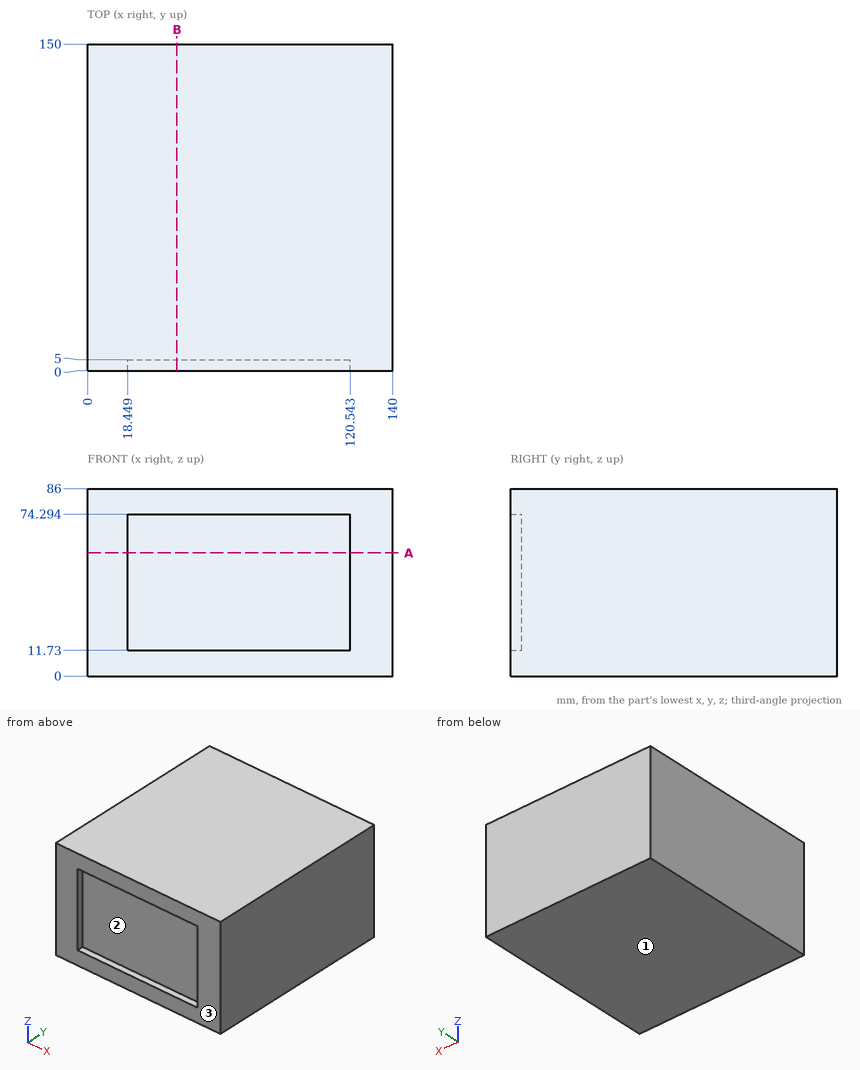
Here's the drawing with two shaded views (mm, measured from the low corner). I have some questions. Coordinates: 2 decimals unless noted, no trailing zeros. Write each loop counter-clockwise with the first axis right and the second up, starting at its lowest first coordinate (ties: lowest second). Pieces come first, ordered by that corner, then holes.
Item 1: If we mould it in two halves opening along Z, with no side actions, what happens to the marked faces 1, 2 and 3? For each: +Z half, -Z half, draft (parallel to the pull), parting line (faces both ways), or undercut.
Item 2: I want a section at A-A on z = 56.5. Write out the boundary of the cut face in (x, y).
Item 3: If I drill on line 1 (Y direction, x = 94, z = 15.5), over which ranges is the centre line in solid material (lowest first)?
Item 4: Will this pin go through, and if not, where does the flat tip stop? pin 1 (8 mm diameter, centred on x = 31.5, z = 39, fed in from -Y).
Item 5: I want a section at B-B on x = 41. Write out the boundary of the cut face in (y, z) (1 decimal), and give its area (3 significant figures).
Findings below:
1. face 1: -Z half
1. face 2: undercut
1. face 3: draft
2. outline: (0, 0) - (18.45, 0) - (18.45, 5) - (120.54, 5) - (120.54, 0) - (140, 0) - (140, 150) - (0, 150) - close
3. line 1: y = 5 to 150
4. pin 1: stops at y = 5
5. outline: (0, 0) - (150, 0) - (150, 86) - (0, 86) - (0, 74.3) - (5, 74.3) - (5, 11.7) - (0, 11.7) - close
5. area: 12,600 mm2
